from build123d import *

# Parameters (mm, degrees)
SKETCH1_R           = 1.5
SKETCH1_R_2         = 41.5
SKETCH1_R_3         = 2.65
SKETCH1_R_4         = 1.65
SKETCH1_R_5         = 1.25
BOSS_EXTRUDE1_DEPTH = 5


with BuildPart() as part:
    # Sketch1 → Boss-Extrude1 (new body)
    with BuildSketch(Plane.XZ):
        with BuildLine():
            Line((159, -192), (325, -192))
            ThreePointArc((325, -192), (328.535533906, -190.535533906), (330, -187))
            Line((330, -187), (330, -160))
            ThreePointArc((330, -160), (328.828427125, -157.171572875), (326, -156))
            Line((326, -156), (306, -156))
            ThreePointArc((306, -156), (303.171572875, -154.828427125), (302, -152))
            Line((302, -152), (302, -144.5))
            ThreePointArc((302, -144.5), (300.828427125, -141.671572875), (298, -140.5))
            Line((298, -140.5), (271, -140.5))
            ThreePointArc((271, -140.5), (268.171572875, -139.328427125), (267, -136.5))
            Line((267, -136.5), (267, -55.5))
            ThreePointArc((267, -55.5), (268.171572875, -52.671572875), (271, -51.5))
            Line((271, -51.5), (298, -51.5))
            ThreePointArc((298, -51.5), (300.828427125, -50.328427125), (302, -47.5))
            Line((302, -47.5), (302, -40))
            ThreePointArc((302, -40), (303.171572875, -37.171572875), (306, -36))
            Line((306, -36), (326, -36))
            ThreePointArc((326, -36), (328.828427125, -34.828427125), (330, -32))
            Line((330, -32), (330, -5))
            ThreePointArc((330, -5), (328.535533906, -1.464466094), (325, 0))
            Line((325, 0), (159, 0))
            ThreePointArc((159, 0), (155.464466094, -1.464466094), (154, -5))
            Line((154, -5), (154, -25))
            ThreePointArc((154, -25), (152.535533906, -28.535533906), (149, -30))
            Line((149, -30), (61, -30))
            ThreePointArc((61, -30), (57.464466094, -28.535533906), (56, -25))
            Line((56, -25), (56, -5))
            ThreePointArc((56, -5), (54.535533906, -1.464466094), (51, 0))
            Line((51, 0), (5, 0))
            ThreePointArc((5, 0), (1.464466094, -1.464466094), (0, -5))
            Line((0, -5), (0, -32))
            ThreePointArc((0, -32), (1.171572875, -34.828427125), (4, -36))
            Line((4, -36), (24, -36))
            ThreePointArc((24, -36), (26.828427125, -37.171572875), (28, -40))
            Line((28, -40), (28, -152))
            ThreePointArc((28, -152), (26.828427125, -154.828427125), (24, -156))
            Line((24, -156), (4, -156))
            ThreePointArc((4, -156), (1.171572875, -157.171572875), (0, -160))
            Line((0, -160), (0, -187))
            ThreePointArc((0, -187), (1.464466094, -190.535533906), (5, -192))
            Line((5, -192), (51, -192))
            ThreePointArc((51, -192), (54.535533906, -190.535533906), (56, -187))
            Line((56, -187), (56, -167))
            ThreePointArc((56, -167), (57.464466094, -163.464466094), (61, -162))
            Line((61, -162), (149, -162))
            ThreePointArc((149, -162), (152.535533906, -163.464466094), (154, -167))
            Line((154, -167), (154, -187))
            ThreePointArc((154, -187), (155.464466094, -190.535533906), (159, -192))
        make_face()
        with Locations(Location((92.587903827, -138.036518729, 0), (0, 0, 90))):
            Circle(SKETCH1_R, mode=Mode.SUBTRACT)
        with Locations(Location((127.412096173, -138.036518729, 0), (0, 0, 90))):
            Circle(SKETCH1_R, mode=Mode.SUBTRACT)
        with Locations(Location((152.036518729, -113.412096173, 0), (0, 0, 90))):
            Circle(SKETCH1_R, mode=Mode.SUBTRACT)
        with Locations(Location((152.036518729, -78.587903827, 0), (0, 0, 90))):
            Circle(SKETCH1_R, mode=Mode.SUBTRACT)
        with Locations(Location((127.412096173, -53.963481271, 0), (0, 0, 90))):
            Circle(SKETCH1_R, mode=Mode.SUBTRACT)
        with Locations(Location((92.587903827, -53.963481271, 0), (0, 0, 90))):
            Circle(SKETCH1_R, mode=Mode.SUBTRACT)
        with Locations(Location((67.963481271, -78.587903827, 0), (0, 0, 90))):
            Circle(SKETCH1_R, mode=Mode.SUBTRACT)
        with Locations(Location((67.963481271, -113.412096173, 0), (0, 0, 90))):
            Circle(SKETCH1_R, mode=Mode.SUBTRACT)
        with Locations(Location((110, -96, 0), (0, 0, 90))):
            Circle(SKETCH1_R_2, mode=Mode.SUBTRACT)
        with Locations(Location((320, -172, 0), (0, 0, 90))):
            Circle(SKETCH1_R_3, mode=Mode.SUBTRACT)
        with Locations(Location((320, -10, 0), (0, 0, 90))):
            Circle(SKETCH1_R_3, mode=Mode.SUBTRACT)
        with Locations(Location((10, -10, 0), (0, 0, 90))):
            Circle(SKETCH1_R_3, mode=Mode.SUBTRACT)
        with Locations(Location((10, -172, 0), (0, 0, 90))):
            Circle(SKETCH1_R_3, mode=Mode.SUBTRACT)
        with Locations(Location((110, -143.5, 0), (0, 0, 90))):
            Circle(SKETCH1_R_4, mode=Mode.SUBTRACT)
        with Locations(Location((62.5, -96, 0), (0, 0, 90))):
            Circle(SKETCH1_R_4, mode=Mode.SUBTRACT)
        with Locations(Location((110, -48.5, 0), (0, 0, 90))):
            Circle(SKETCH1_R_4, mode=Mode.SUBTRACT)
        with Locations(Location((157.5, -96, 0), (0, 0, 90))):
            Circle(SKETCH1_R_4, mode=Mode.SUBTRACT)
        with Locations(Location((202.5, -126.310889132, 0), (0, 0, 90))):
            Circle(SKETCH1_R_5, mode=Mode.SUBTRACT)
        with Locations(Location((255, -96, 0), (0, 0, 90))):
            Circle(SKETCH1_R_5, mode=Mode.SUBTRACT)
        with Locations(Location((202.5, -65.689110868, 0), (0, 0, 90))):
            Circle(SKETCH1_R_5, mode=Mode.SUBTRACT)
        with Locations(Location((156, -46.5, 0), (0, 0, 90))):
            Circle(SKETCH1_R_5, mode=Mode.SUBTRACT)
        with Locations(Location((174, -46.5, 0), (0, 0, 90))):
            Circle(SKETCH1_R_5, mode=Mode.SUBTRACT)
        with BuildLine():
            ThreePointArc((210.22518928, -59.796366544), (238.75, -63.524047358), (256.240671642, -86.363417673))
            ThreePointArc((256.240671642, -86.363417673), (255.870910902, -89.335183714), (253.541666667, -91.217399882))
            ThreePointArc((253.541666667, -91.217399882), (250, -96), (253.541666667, -100.782600118))
            ThreePointArc((253.541666667, -100.782600118), (255.870910902, -102.664816286), (256.240671642, -105.636582327))
            ThreePointArc((256.240671642, -105.636582327), (238.75, -128.475952642), (210.22518928, -132.203633456))
            ThreePointArc((210.22518928, -132.203633456), (207.836444764, -130.397528241), (207.371019865, -127.439235478))
            ThreePointArc((207.371019865, -127.439235478), (205, -121.980762114), (199.087313468, -122.65663536))
            ThreePointArc((199.087313468, -122.65663536), (196.292644334, -123.732711955), (193.534139078, -122.567051128))
            ThreePointArc((193.534139078, -122.567051128), (182.5, -96), (193.534139078, -69.432948872))
            ThreePointArc((193.534139078, -69.432948872), (196.292644334, -68.267288045), (199.087313468, -69.34336464))
            ThreePointArc((199.087313468, -69.34336464), (205, -70.019237886), (207.371019865, -64.560764522))
            ThreePointArc((207.371019865, -64.560764522), (207.836444764, -61.602471759), (210.22518928, -59.796366544))
        make_face(mode=Mode.SUBTRACT)
    extrude(amount=-BOSS_EXTRUDE1_DEPTH)


solid = part.part
Design review of the part built by this model. Coordinates are the model's own, in mm. A direction names the side the tool comes from. Coordinates: 2 decimals unless noted, no trailing zeros. Use CSV: the item, a comma, the result in double quotes. Start each with the question number.
1. Add section A-A on y = 1.5. Count the separate pieces of the cut face and the enclosed holes in it, plus the area to 3 significant figures.
2. Clearance check with flat-ended pins moving along their axes: pin 1 (3 mm diameter, centred on x = 120.5, y = 4, fed in from +Z); pin 2 (3 mm diameter, centred on y = 2.5, z = -88, fed in from +X). State where each tip first meets the part, or that it passes through.
3. For faces 3 (the cylindrical face through (238.39, 2.46, -63.32)), 4 (the flat face through (163, 5, -95)), list the 3-axis set-ups (+Z, -Z, +X, -X, +Y, -Y) from which the entire face can be reached by the end or side of a thin tool; tool diameter is ignored.
4. To check wall thickness, follow probe 1 along X at (y, z) = (2.65, -96); probe 2 along X at (y, z) = (3.3, -10); probe 3 along X at (y, z) = (3.25, -16). State the ranges of each line that lie inside material, in increasing order.
5. Mouldability with a two-part tool opening along X and no side actions: class faces 1 (the cylindrical face through (239.107, 2.465, -128.267)), 2 (the flat face through (163, 0, -95)) as released by +X, released by -X, zero draft, split by the parting line, or undercut.
Resolved:
1,separate pieces,"1"
1,enclosed holes,"23"
1,area,"37,800 mm2"
2,pin 1,"z = -30"
2,pin 2,"x = 267"
3,face 3,"+Y, -Y"
3,face 4,"+Z, -Z, +X, -X, +Y"
4,probe 1,"28 to 60.85, 64.15 to 68.5, 151.5 to 155.85, 159.15 to 182.5, 250 to 253.75, 256.25 to 267"
4,probe 2,"0 to 7.35, 12.65 to 56, 154 to 317.35, 322.65 to 330"
4,probe 3,"0 to 56, 154 to 330"
5,face 1,"undercut"
5,face 2,"zero draft"
